```python
from build123d import *

# Parameters (mm, degrees)
ESQUISSE1_W             = 102
ESQUISSE1_H             = 60
BOSS_EXTRU_1_DEPTH      = 8.1
ESQUISSE2_R             = 1.75
ENL_V_MAT_EXTRU_1_DEPTH = 119.61538686
ESQUISSE5_W             = 51.9
ESQUISSE5_H             = 8
BOSS_EXTRU_2_DEPTH      = 8.1
ESQUISSE6_W             = 16
ESQUISSE6_H             = 20
ENL_V_MAT_EXTRU_2_DEPTH = 119.61538686
CONG_1_R                = 3


with BuildPart() as part:
    # Esquisse1 → Boss.-Extru.1 (new body)
    with BuildSketch(Plane.XY):
        with Locations((51, 30)):
            Rectangle(ESQUISSE1_W, ESQUISSE1_H)
    extrude(amount=BOSS_EXTRU_1_DEPTH)

    # Esquisse2 → Enlèv. mat.-Extru.1 (cut, through all)
    with BuildSketch(Plane.XY.offset(8.1)):
        with Locations((4, 55)):
            Circle(ESQUISSE2_R)
        with Locations((4, 31)):
            Circle(ESQUISSE2_R)
        with Locations((98, 24)):
            Circle(ESQUISSE2_R)
        with Locations((98, 4)):
            Circle(ESQUISSE2_R)
        with Locations(Location((59.9, 4, 0), (0, 0, 180))):
            Circle(ESQUISSE2_R)
        with Locations(Location((59.9, 24, 0), (0, 0, 180))):
            Circle(ESQUISSE2_R)
        with Locations(Location((42.1, 31, 0), (0, 0, 180))):
            Circle(ESQUISSE2_R)
        with Locations(Location((42.1, 55, 0), (0, 0, 180))):
            Circle(ESQUISSE2_R)
        with Locations((66.95, 7.5)):
            Circle(ESQUISSE2_R)
        with Locations((78.95, 7.5)):
            Circle(ESQUISSE2_R)
        with Locations(Location((90.95, 7.5, 0), (0, 0, 180))):
            Circle(ESQUISSE2_R)
    extrude(amount=-ENL_V_MAT_EXTRU_1_DEPTH, mode=Mode.SUBTRACT)

    # Esquisse5 → Boss.-Extru.2 (add)
    with BuildSketch(Plane.XY.offset(8.1)):
        with Locations((25.95, -4)):
            Rectangle(ESQUISSE5_W, ESQUISSE5_H)
    extrude(amount=-BOSS_EXTRU_2_DEPTH)

    # Esquisse6 → Enlèv. mat.-Extru.2 (cut, through all)
    with BuildSketch(Plane.XY.offset(8.1)):
        with Locations((23.05, 35)):
            Rectangle(ESQUISSE6_W, ESQUISSE6_H)
        with Locations((78.95, 26)):
            Rectangle(ESQUISSE6_W, ESQUISSE6_H)
    extrude(amount=-ENL_V_MAT_EXTRU_2_DEPTH, mode=Mode.SUBTRACT)

    # Congé1
    cong_1_edges = [part.edges().sort_by_distance(p)[0] for p in [
        (15.05, 25, 4.05),
        (15.05, 45, 4.05),
        (31.05, 45, 4.05),
        (31.05, 25, 4.05),
        (86.95, 36, 4.05),
        (86.95, 16, 4.05),
        (70.95, 16, 4.05),
        (70.95, 36, 4.05),
    ]]
    fillet(cong_1_edges, radius=CONG_1_R)


solid = part.part
```
Check sheet for the modelled part. Datum: model origin and axes. Units: mm. Round coordinates to 2 decimals unless told otherwise and drop trailing zeros. Loops run counter-clockwise (first coordinate to the right, second up) from the corner with the lowest first, then second, coordinate; pieces in that order, holes last. Notation, with made-up numbers: (51, -3) -> (91, -3) arc R12 ccw to (91, 10) -> close; hole circle Ø4 at (50.5, 15.25). An arc over 180 degrees is marked (long way). Answer in a Markdown table with one row per item.
Q1. Sectioned sample at B-B on x = 66.95. Enter the section's corners in (y, z).
Data:
| item | result |
|---|---|
| outline | (0, 0) -> (5.75, 0) -> (5.75, 8.1) -> (0, 8.1) -> close; (9.25, 0) -> (60, 0) -> (60, 8.1) -> (9.25, 8.1) -> close |
Q2. Sectioned sample at D-D on z = 6.5. Give the number of separate pieces and of enclosed holes in the cut face, then the cut area to 3 significant figures.
Data:
| item | result |
|---|---|
| separate pieces | 1 |
| enclosed holes | 13 |
| area | 5,800 mm^2 |
Q3. Go/stop test with flat-tipped pins: P1, Ø2, axis at x = 59.9, y = 24, coming from the +Z side; P2, Ø4, axis at x = 69, z = 5.5, coming from the -Y side. Record where each tip stops, or that it passes through.
Data:
| item | result |
|---|---|
| P1 | passes through |
| P2 | stops at y = 0 |
Q4. Thickness scan on L1, parallel to Y at x = 42.1, z = 5.25; L2, parallel to Y at x = 81.5, z = 3.5; L3, parallel to X at y = 30.5, z = 3.25. Record the ranges inside material, lowest first.
Data:
| item | result |
|---|---|
| L1 | y = -8 to 29.25, 32.75 to 53.25, 56.75 to 60 |
| L2 | y = 0 to 16, 36 to 60 |
| L3 | x = 0 to 2.32, 5.68 to 15.05, 31.05 to 40.42, 43.78 to 70.95, 86.95 to 102 |
Q5. Sectioned sample at C-C on y = 55. Enter the section's corners in (x, z), then the cut area to 4 significant figures.
Data:
| item | result |
|---|---|
| outline | (0, 0) -> (2.25, 0) -> (2.25, 8.1) -> (0, 8.1) -> close; (5.75, 0) -> (40.35, 0) -> (40.35, 8.1) -> (5.75, 8.1) -> close; (43.85, 0) -> (102, 0) -> (102, 8.1) -> (43.85, 8.1) -> close |
| area | 769.5 mm^2 |
Q6. Sectioned sample at A-A on x = 4. Enter the section's corners in (y, z), then the cut area to 3 significant figures.
Data:
| item | result |
|---|---|
| outline | (-8, 0) -> (29.25, 0) -> (29.25, 8.1) -> (-8, 8.1) -> close; (32.75, 0) -> (53.25, 0) -> (53.25, 8.1) -> (32.75, 8.1) -> close; (56.75, 0) -> (60, 0) -> (60, 8.1) -> (56.75, 8.1) -> close |
| area | 494 mm^2 |
Q7. Release check for a two-part mould opening along X. For faces 1 (the face through (50, 26, 0)), 2 (the face through (79, 16, 4)), 3 (the face through (0, 26, 4)), 4 (the face through (102, 30, 4)) record: released by +X, released by -X, zero draft, split by the parting line, or undercut.
Data:
| item | result |
|---|---|
| face 1 | zero draft |
| face 2 | undercut |
| face 3 | released by -X |
| face 4 | released by +X |
